```python
from build123d import *

# Parameters (mm, degrees)
ESQUISSE1_W        = 30
ESQUISSE1_H        = 30
ESQUISSE1_R        = 2.5
BOSS_EXTRU_1_DEPTH = 7
ESQUISSE2_W        = 6
ESQUISSE2_H        = 1
BOSS_EXTRU_2_DEPTH = 15


with BuildPart() as part:
    # Esquisse1 → Boss.-Extru.1 (new body)
    with BuildSketch(Plane.XY):
        with Locations((11.780048077, -12.282786885)):
            Rectangle(ESQUISSE1_W, ESQUISSE1_H)
        with Locations((11.780048077, -12.282786885)):
            Circle(ESQUISSE1_R, mode=Mode.SUBTRACT)
    extrude(amount=BOSS_EXTRU_1_DEPTH)

    # Esquisse2 → Boss.-Extru.2 (add)
    with BuildSketch(Plane.XY.offset(7)):
        with Locations((4.780048077, -2.782786885)):
            Rectangle(ESQUISSE2_W, ESQUISSE2_H)
        with Locations((18.780048077, -2.782786885)):
            Rectangle(ESQUISSE2_W, ESQUISSE2_H)
        with Locations((4.780048077, -21.782786885)):
            Rectangle(ESQUISSE2_W, ESQUISSE2_H)
        with Locations((18.780048077, -21.782786885)):
            Rectangle(ESQUISSE2_W, ESQUISSE2_H)
    extrude(amount=BOSS_EXTRU_2_DEPTH)


solid = part.part
```
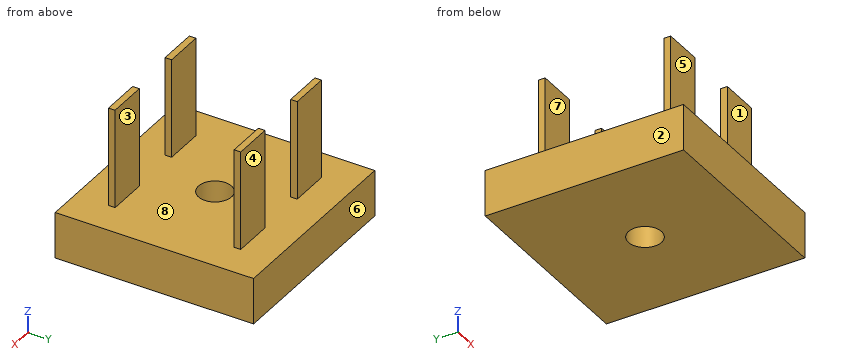
Geometry: final body of the model. Coordinates: model frame, mm. Face numbers are marked on the shaded views. A direction names the side the tool comes from. Round coordinates to 2 decimals unless told otherwise and drop trailing zeros. Loops run counter-clockwise (first coordinate to the right, second up) from the corner with the lowest first, then second, coordinate; pieces in that order, holes last. Notation, with made-up numbers: (-15.5, 38.25) -> (-11.5, 38.25) arc R29 cw to (-11.5, 65.25) -> close; hole circle Ø4 at (23.25, 75.5). An arc over 180 degrees is marked (long way). Write each question's results on one line, items separated by ' | '.
Item 1: Pull-direction query (Y, two-part tool) for the marked faces 5, 6, 7 and 8; classes: pulls with the +Y half, pulls with the -Y half, needs draft (parallel to the pull), parting line crosses it, or undercut.
Answers below:
face 5: pulls with the -Y half | face 6: pulls with the +Y half | face 7: undercut | face 8: undercut
Item 2: Cut plane C-C on x = 5.5. Return the cut outline in (y, z), and give its area (3 significant figures).
Answers below:
outline: (-27.28, 0) -> (2.72, 0) -> (2.72, 7) -> (-2.28, 7) -> (-2.28, 22) -> (-3.28, 22) -> (-3.28, 7) -> (-21.28, 7) -> (-21.28, 22) -> (-22.28, 22) -> (-22.28, 7) -> (-27.28, 7) -> close | area: 240 mm²
Item 3: Cut plane D-D on x = 13.5. Return the cut outline in (y, z), and give its area (3 significant figures).
Answers below:
outline: (-27.28, 0) -> (-14.1, 0) -> (-14.1, 7) -> (-27.28, 7) -> close; (-10.47, 0) -> (2.72, 0) -> (2.72, 7) -> (-10.47, 7) -> close | area: 185 mm²
Item 4: Cut plane A-A on z = 10. Return the cut outline in (x, y), and give its area (3 significant figures).
Answers below:
outline: (1.78, -22.28) -> (7.78, -22.28) -> (7.78, -21.28) -> (1.78, -21.28) -> close; (1.78, -3.28) -> (7.78, -3.28) -> (7.78, -2.28) -> (1.78, -2.28) -> close; (15.78, -22.28) -> (21.78, -22.28) -> (21.78, -21.28) -> (15.78, -21.28) -> close; (15.78, -3.28) -> (21.78, -3.28) -> (21.78, -2.28) -> (15.78, -2.28) -> close | area: 24.0 mm²
Item 5: Set-up query: the marked faces 1, 2, 3 and 4. Return all of +Z, -Z, +X, -X, +Y, -Y with unobstructed straight access to the full face (end or side cutting, diameter ignored); none if empty.
Answers below:
face 1: +Z, +X, -X, -Y | face 2: +Z, -Z, -X, +Y, -Y | face 3: +Z, +X, -X | face 4: +Z, +X, -X, +Y
Item 6: Cut plane B-B on y = -12.75. Return the cut outline in (x, z), and give its area (3 significant figures).
Answers below:
outline: (-3.22, 0) -> (9.32, 0) -> (9.32, 7) -> (-3.22, 7) -> close; (14.24, 0) -> (26.78, 0) -> (26.78, 7) -> (14.24, 7) -> close | area: 176 mm²
Item 7: Line query: probe 1 along Y at (x, z) = (7.5, 20); probe 2 along Z at (x, y) = (8.5, -8); probe 3 along X at (y, z) = (-2.5, 12). Output: solid intervals per line, ascending. Write a range as [from, to].
Answers below:
probe 1: y = [-22.28, -21.28], [-3.28, -2.28] | probe 2: z = [0, 7] | probe 3: x = [1.78, 7.78], [15.78, 21.78]
Item 8: Pin query (flat end, axial travel): pin 1 Ø1.1 at (y, z) = (-3, 14) entering from -X; pin 2 Ø3 at (x, z) = (3.5, 16) entering from +Y; pin 3 Ø2 at (x, z) = (22.5, 8.5) entering from -Y. Return the tip coordinate at first contact, or that it passes through.
Answers below:
pin 1: stops at x = 1.78 | pin 2: stops at y = -2.28 | pin 3: stops at y = -22.28
